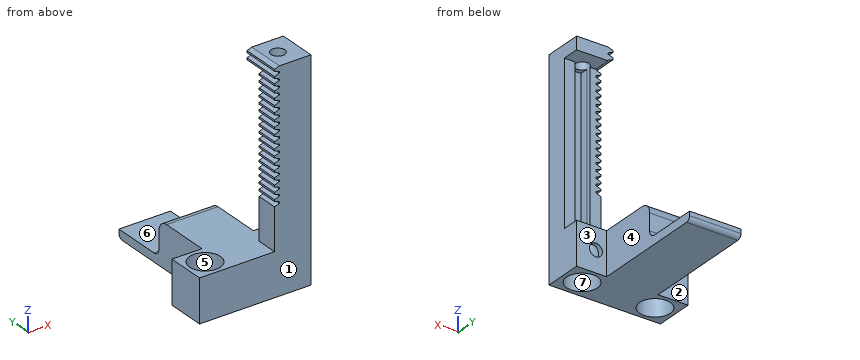
from build123d import *

# Parameters (mm, degrees)
SKETCH_1_W             = 26
SKETCH_1_H             = 9
EXTRUDE_1_DEPTH        = 10
SKETCH_2_R             = 3.6
CUT_EXTRUDE_1_DEPTH    = 18.007351352
EXTRUDE_2_DEPTH        = 26
CUT_EXTRUDE_2_DEPTH    = 7
SKETCH_7_W             = 8.5
SKETCH_7_H             = 9
EXTRUDE_3_DEPTH        = 40
SKETCH_8_R             = 1.6
CUT_EXTRUDE_3_DEPTH    = 40
SKETCH_9_W             = 3.5
SKETCH_9_H             = 37
CUT_EXTRUDE_4_DEPTH    = 7
CUT_EXTRUDE_12_DEPTH   = 50.979995998
PATTERN_START          = -4.5
PATTERN_LINEAR_2_DEPTH = 9
SKETCH_22_W            = 8.5
SKETCH_22_H            = 37
CUT_EXTRUDE_13_DEPTH   = 4
SKETCH_23_R            = 1.5
CUT_EXTRUDE_14_DEPTH   = 4


# Read off the part's stored shape, not the designer's step: 阵列(线性)2
with BuildPart() as part:
    # 草图1 → 凸台-拉伸1 (new body)
    with BuildSketch(Plane.XY):
        Rectangle(SKETCH_1_W, SKETCH_1_H)
    extrude(amount=-EXTRUDE_1_DEPTH)

    # 草图2 → 切除-拉伸1 (cut, through all)
    with BuildSketch(Plane.XY):
        with Locations((8.5, 0)):
            Circle(SKETCH_2_R)
        with Locations(Location((-8.5, 0, 0), (0, 0, 180))):
            Circle(SKETCH_2_R)
    extrude(amount=-CUT_EXTRUDE_1_DEPTH, mode=Mode.SUBTRACT)

    # 草图5 → 凸台-拉伸2 (add, through all)
    with BuildSketch(Plane.ZY.offset(13)):
        with BuildLine():
            Line((0, 4.5), (-10, 4.5))
            Line((-10, 4.5), (-10, 8.301419967))
            Line((-10, 8.301419967), (-10, 30.5))
            ThreePointArc((-10, 30.5), (-9.707106781, 31.207106781), (-9, 31.5))
            Line((-9, 31.5), (-8, 31.5))
            Line((-8, 31.5), (-8, 20.1))
            ThreePointArc((-8, 20.1), (-7.53137085, 18.96862915), (-6.4, 18.5))
            Line((-6.4, 18.5), (-2.5, 18.5))
            ThreePointArc((-2.5, 18.5), (-0.732233047, 17.767766953), (0, 16))
            Line((0, 16), (0, 4.5))
        make_face()
    extrude(amount=-EXTRUDE_2_DEPTH)

    # 草图5<2> → 切除-拉伸2 (cut)
    with BuildSketch(Plane.ZY.offset(13)):
        with BuildLine():
            Line((0, 4.5), (-10, 4.5))
            Line((-10, 4.5), (-10, 8.301419967))
            Line((-10, 8.301419967), (-10, 30.5))
            ThreePointArc((-10, 30.5), (-9.707106781, 31.207106781), (-9, 31.5))
            Line((-9, 31.5), (-8, 31.5))
            Line((-8, 31.5), (-8, 20.1))
            ThreePointArc((-8, 20.1), (-7.53137085, 18.96862915), (-6.4, 18.5))
            Line((-6.4, 18.5), (-2.5, 18.5))
            ThreePointArc((-2.5, 18.5), (-0.732233047, 17.767766953), (0, 16))
            Line((0, 16), (0, 4.5))
        make_face()
    cut_extrude_2 = extrude(amount=-CUT_EXTRUDE_2_DEPTH, mode=Mode.SUBTRACT)

    # 镜向1: 切除-拉伸2 across plane
    add(cut_extrude_2.mirror(Plane(origin=(0, 0, 0), x_dir=(0, 0, 1), z_dir=(1, 0, 0))), mode=Mode.SUBTRACT)

    # 草图7 → 凸台-拉伸3 (add)
    with BuildSketch(Plane.XY):
        with Locations((8.75, 0)):
            Rectangle(SKETCH_7_W, SKETCH_7_H)
    extrude(amount=EXTRUDE_3_DEPTH)

    # 草图8 → 切除-拉伸3 (cut)
    with BuildSketch(Plane.XY.offset(40)):
        with Locations((8.5, 0)):
            Circle(SKETCH_8_R)
    extrude(amount=-CUT_EXTRUDE_3_DEPTH, mode=Mode.SUBTRACT)

    # 草图9 → 切除-拉伸4 (cut)
    with BuildSketch(Plane(origin=(0, 4.5, 0), x_dir=(1, 0, 0), z_dir=(0, 1, 0))):
        with Locations((8.75, -18.5)):
            Rectangle(SKETCH_9_W, SKETCH_9_H)
    extrude(amount=-CUT_EXTRUDE_4_DEPTH, mode=Mode.SUBTRACT)

    # 草图10 → 切除-拉伸12 (cut, through all)
    with BuildSketch(Plane(origin=(0, 4.5, 0), x_dir=(1, 0, 0), z_dir=(0, 1, 0))):
        Polygon((5.625, -40), (5.625, -40.330435371), (4.5, -40.739901884), (4.5, -39.590533486), align=None)
    extrude(amount=-CUT_EXTRUDE_12_DEPTH, mode=Mode.SUBTRACT)

    # 阵列(线性)2 outline → 阵列(线性)2 (cut)
    with BuildSketch(Plane(origin=(0, 0, 0), x_dir=(1, 0, 0), z_dir=(0, 1, 0)).offset(PATTERN_START)):
        Polygon((5.625, -10.485305161), (5.625, -10.154869791), (4.5, -9.745403277), (4.5, -10.894771675), align=None)
        Polygon((5.625, -38.429203673), (4.5, -38.01973716), (4.5, -39.169105557), (5.625, -38.759639044), align=None)
        Polygon((5.625, -36.858407346), (4.5, -36.448940833), (4.5, -37.598309231), (5.625, -37.188842717), align=None)
        Polygon((5.625, -35.28761102), (4.5, -34.878144506), (4.5, -36.027512904), (5.625, -35.61804639), align=None)
        Polygon((5.625, -33.716814693), (4.5, -33.307348179), (4.5, -34.456716577), (5.625, -34.047250063), align=None)
        Polygon((5.625, -32.146018366), (4.5, -31.736551852), (4.5, -32.88592025), (5.625, -32.476453737), align=None)
        Polygon((5.625, -30.575222039), (4.5, -30.165755526), (4.5, -31.315123923), (5.625, -30.90565741), align=None)
        Polygon((5.625, -29.004425712), (4.5, -28.594959199), (4.5, -29.744327597), (5.625, -29.334861083), align=None)
        Polygon((5.625, -27.433629386), (4.5, -27.024162872), (4.5, -28.17353127), (5.625, -27.764064756), align=None)
        Polygon((5.625, -25.862833059), (4.5, -25.453366545), (4.5, -26.602734943), (5.625, -26.193268429), align=None)
        Polygon((5.625, -24.292036732), (4.5, -23.882570219), (4.5, -25.031938616), (5.625, -24.622472103), align=None)
        Polygon((5.625, -22.721240405), (4.5, -22.311773892), (4.5, -23.461142289), (5.625, -23.051675776), align=None)
        Polygon((5.625, -21.150444078), (4.5, -20.740977565), (4.5, -21.890345963), (5.625, -21.480879449), align=None)
        Polygon((5.625, -19.579647752), (4.5, -19.170181238), (4.5, -20.319549636), (5.625, -19.910083122), align=None)
        Polygon((5.625, -18.008851425), (4.5, -17.599384911), (4.5, -18.748753309), (5.625, -18.339286795), align=None)
        Polygon((5.625, -16.438055098), (4.5, -16.028588585), (4.5, -17.177956982), (5.625, -16.768490469), align=None)
        Polygon((5.625, -14.867258771), (4.5, -14.457792258), (4.5, -15.607160655), (5.625, -15.197694142), align=None)
        Polygon((5.625, -13.296462444), (4.5, -12.886995931), (4.5, -14.036364329), (5.625, -13.626897815), align=None)
        Polygon((5.625, -11.725666118), (4.5, -11.316199604), (4.5, -12.465568002), (5.625, -12.056101488), align=None)
    extrude(amount=PATTERN_LINEAR_2_DEPTH, mode=Mode.SUBTRACT)

    # 草图22 → 切除-拉伸13 (cut)
    with BuildSketch(Plane(origin=(0, 4.5, 0), x_dir=(1, 0, 0), z_dir=(0, 1, 0))):
        with Locations((8.75, -18.5)):
            Rectangle(SKETCH_22_W, SKETCH_22_H)
    extrude(amount=-CUT_EXTRUDE_13_DEPTH, mode=Mode.SUBTRACT)

    # 草图23 → 切除-拉伸14 (cut)
    with BuildSketch(Plane(origin=(0, 4.5, 0), x_dir=(1, 0, 0), z_dir=(0, 1, 0))):
        with Locations(Location((8.5, 5, 0), (0, 0, 270))):
            Circle(SKETCH_23_R)
        with Locations(Location((-8.5, 5, 0), (0, 0, 270))):
            Circle(SKETCH_23_R)
    extrude(amount=-CUT_EXTRUDE_14_DEPTH, mode=Mode.SUBTRACT)


solid = part.part
Work out the finished part from the listing and answer in its coordinate system (mm). Face numbers are marked on the shaded views. A direction names the side the tool comes from. Round coordinates to 2 decimals unless told otherwise and drop trailing zeros. Write each loop counter-clockwise with the first axis right and the second up, starting at its lowest first coordinate (ties: lowest second). Pieces come first, ordered by that corner, then holes. Notation, with made-up numbers: (74.25, -16.75) -> (131.25, -16.75) arc R15 cw to (131.25, 4.25) -> close; hole circle Ø9 at (80.25, 7.5). An arc over 180 degrees is marked (long way). Answer as CSV lines item,"result". Start each with the question number.
(1) The mould has two halves that part along X. Classify the marked faces 4, 5, 6 and 7: +X half, -X half, draft (parallel to the pull), parting line (faces both ways), or undercut.
(2) Each of these flat-tipped pins is pushed along its axis until it touches: pin 1 (0.7 mm diameter, centred on x = 5.5, z = 10, fed in from +Y); pin 2 (1.5 mm diameter, centred on x = -1, y = 25, fed in from +Z); pin 3 (0.5 mm diameter, centred on y = -1.5, z = 14, fed in from -X). Where does it stop, or does it pass through?
(3) The part is cut by section B-B, the plane z = -5. Give the vertices of the cut face in (x, y), then the cut area to 3 significant figures.
(4) A tool of negligible diameter and unlimited length cuts with its end or side. For the marked faces 1, 2 and 3, from which of +Z, -Z, +X, -X, +Y, -Y can it reach the whole face along a straight path? Write none if from no direction.
(5) Find the intervals of material crossed by probe 1 along X at (y, z) = (4.1, -5); probe 2 along Z at (x, y) = (8.5, 4.15); probe 3 along X at (y, z) = (0, 28.5), in increasing order.
(6) The part is cut by section D-D, the plane x = -7.75. Give the vertices of the cut face in (y, z).
(7) The part is cut by section C-C, the plane x = -1.5. Give the vertices of the cut face in (y, z).
(8) The part is cut by section A-A, the plane x = 8.5. Give the vertices of the cut face in (y, z).
Output values:
1,face 4,"+X half"
1,face 5,"undercut"
1,face 6,"draft"
1,face 7,"undercut"
2,pin 1,"stops at y = 0.5"
2,pin 2,"stops at z = -8"
2,pin 3,"stops at x = 4.5"
3,outline,"(-13, -4.5) -> (13, -4.5) -> (13, 4.5) -> (10, 4.5) -> (10, 3.27) arc R3.6 cw (long way) to (7, 3.27) -> (7, 4.5) -> (6, 4.5) -> (6, 18.5) -> (-6, 18.5) -> (-6, 4.5) -> (-7, 4.5) -> (-7, 3.27) arc R3.6 cw (long way) to (-10, 3.27) -> (-10, 4.5) -> (-13, 4.5) -> close"
3,area,"315 mm²"
4,face 1,"+Z, -Z, +X, -X, -Y"
4,face 2,"+Z, -Z, -X, +Y"
4,face 3,"+Z, -Z, +X, +Y"
5,probe 1,"x = -13 to -10, -7 to 7, 10 to 13"
5,probe 2,"z = -10 to -6.5, -3.5 to 0, 37 to 40"
5,probe 3,"x = 4.5 to 6.9, 10.5 to 13"
6,outline,"(-4.5, -10) -> (-3.52, -10) -> (-3.52, 0) -> (-4.5, 0) -> close; (3.52, -10) -> (4.5, -10) -> (4.5, -6.3) -> (3.52, -6.3) -> close; (3.52, -3.7) -> (4.5, -3.7) -> (4.5, 0) -> (3.52, 0) -> close"
7,outline,"(-4.5, -10) -> (30.5, -10) arc R1 ccw to (31.5, -9) -> (31.5, -8) -> (20.1, -8) arc R1.6 cw to (18.5, -6.4) -> (18.5, -2.5) arc R2.5 ccw to (16, 0) -> (-4.5, 0) -> close"
8,outline,"(-4.5, -10) -> (-3.6, -10) -> (-3.6, 0) -> (-2.5, 0) -> (-2.5, 37) -> (-1.6, 37) -> (-1.6, 40) -> (-4.5, 40) -> close; (1.6, 37) -> (4.5, 37) -> (4.5, 40) -> (1.6, 40) -> close; (3.6, -10) -> (4.5, -10) -> (4.5, -6.5) -> (3.6, -6.5) -> close; (3.6, -3.5) -> (4.5, -3.5) -> (4.5, 0) -> (3.6, 0) -> close"
